Here's the drawing with two shaded views (mm, measured from the low corner). I have some questions. A direction names the side the tool comes from. Give positions to 0.01 mm unless a question says otherwise; leave off trailing zeros. Order: outer loops, then holes, each group sorted by start corner. A loop starts at its lowest first (then second) coordinate and runs counter-clockwise, first axis right, second up. Notation, with made-up numbers: M 60,-24.75 L 78,-24.75 A8 cw 78,-17.75 Z; hole C 66,-26.5 d3. An arc over 180 degrees is marked long. Write each question's results on one line, items separated by ' | '.
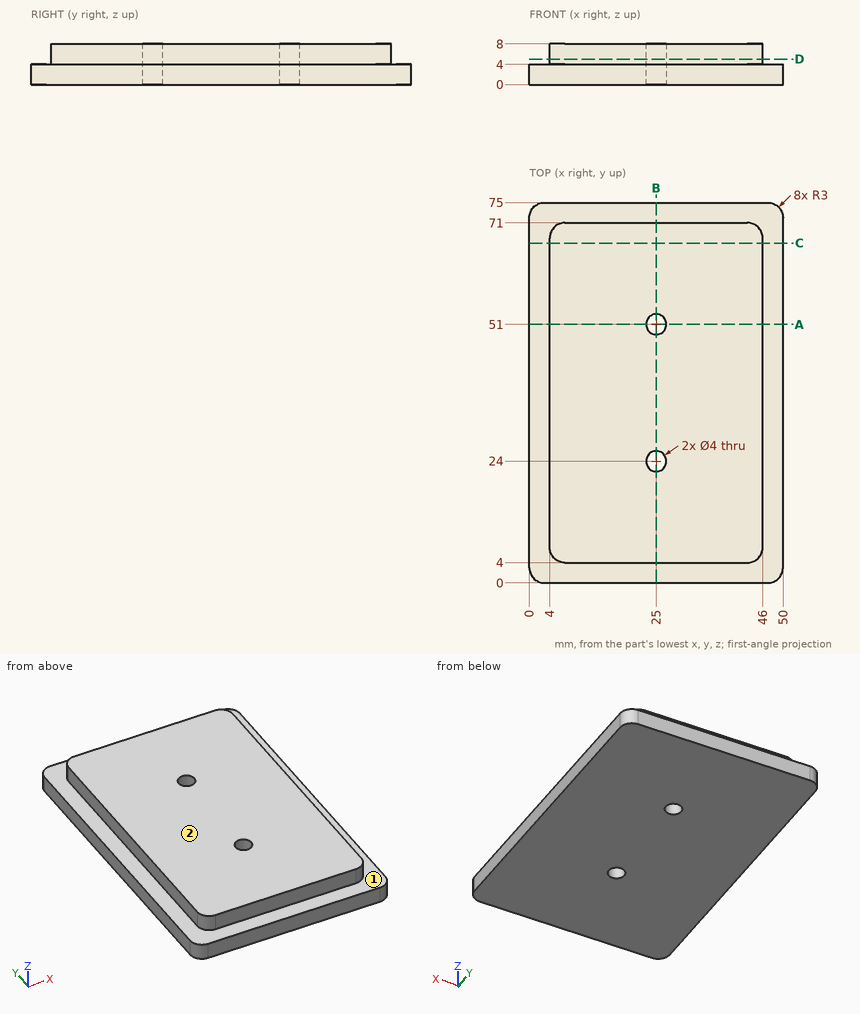
(1) For the marked faces 1 and 2, which set-ups out of +Z, -Z, +X, -X, +Y, -Y let a thin tool reach every point of the face, with its end or its side?
Data:
face 1: +Z | face 2: +Z, +X, -X, +Y, -Y
(2) Imagine slicing it at C-C, the plane y = 67. Write out the boundary of the cut face in (x, z).
Data:
outline: M 0,0 L 50,0 L 50,4 L 46,4 L 46,8 L 4,8 L 4,4 L 0,4 Z
(3) Will these pins go through, and if not, where does the flat tip stop? P1, Ø6.5, axis at x = 25, y = 51, coming from the -Z side; P2, Ø2, axis at x = 23, z = 5.5, coming from the -Y side; P3, Ø2, axis at y = 45, z = 5.5, coming from the +X side; P4, Ø1.5, axis at y = 42.5, z = 6, coming from the -X side.
Data:
P1: stops at z = 0 | P2: stops at y = 4 | P3: stops at x = 46 | P4: stops at x = 4
(4) I need wall thicknesses on L1, parallel to Y at x = 25, z = 2.25; L2, parallel to Y at x = 24.5, z = 0.5; L3, parallel to X at y = 18, z = 6.75. Which ranges of each line are inside material? Lowest first, please. Write a range as from..to.
Data:
L1: y = 0..22, 26..49, 53..75 | L2: y = 0..22.06, 25.94..49.06, 52.94..75 | L3: x = 4..46
(5) Imagine slicing it at B-B, the plane x = 25. Write out the boundary of the cut face in (y, z).
Data:
outline: M 0,0 L 22,0 L 22,8 L 4,8 L 4,4 L 0,4 Z; M 26,0 L 49,0 L 49,8 L 26,8 Z; M 53,0 L 75,0 L 75,4 L 71,4 L 71,8 L 53,8 Z
(6) Imagine slicing it at A-A, the plane y = 51. Write out the boundary of the cut face in (x, z).
Data:
outline: M 0,0 L 23,0 L 23,8 L 4,8 L 4,4 L 0,4 Z; M 27,0 L 50,0 L 50,4 L 46,4 L 46,8 L 27,8 Z
(7) Imagine slicing it at D-D, the plane z = 5. Write out the boundary of the cut face in (x, y), plus the area to 3 significant figures.
Data:
outline: M 4,7 A3 ccw 7,4 L 43,4 A3 ccw 46,7 L 46,68 A3 ccw 43,71 L 7,71 A3 ccw 4,68 Z; hole C 25,24 d4; hole C 25,51 d4 | area: 2,780 mm2
